```python
from build123d import *

# Parameters (mm, degrees)
SKETCH1_W           = 88.9
SKETCH1_H           = 114.3
BOSS_EXTRUDE1_DEPTH = 5.334
SKETCH2_W           = 5.334
SKETCH2_H           = 16.328571428
CUT_EXTRUDE1_DEPTH  = 6.334
SKETCH2_2_W         = 5.334
SKETCH2_2_H         = 16.328571428
BOSS_EXTRUDE2_DEPTH = 5.334
SKETCH2_3_W         = 5.334
SKETCH2_3_H         = 16.328571428
CUT_EXTRUDE2_DEPTH  = 6.334
CUT_EXTRUDE3_DEPTH  = 6.334


with BuildPart() as part:
    # Sketch1 → Boss-Extrude1 (new body)
    with BuildSketch(Plane(origin=(0, 0, 0), x_dir=(1, 0, 0), z_dir=(0, 1, 0))):
        Rectangle(SKETCH1_W, SKETCH1_H)
    extrude(amount=BOSS_EXTRUDE1_DEPTH)

    # Sketch2 → Cut-Extrude1 (cut, through all)
    with BuildSketch(Plane(origin=(0, 5.334, 0), x_dir=(1, 0, 0), z_dir=(0, 1, 0))):
        with Locations((41.783, -32.657142857)):
            Rectangle(SKETCH2_W, SKETCH2_H)
        with Locations((41.783, 0)):
            Rectangle(SKETCH2_W, SKETCH2_H)
        with Locations((41.783, 32.657142857)):
            Rectangle(SKETCH2_W, SKETCH2_H)
        with Locations((-41.783, 32.657142857)):
            Rectangle(SKETCH2_W, SKETCH2_H)
        with Locations((-41.783, 0)):
            Rectangle(SKETCH2_W, SKETCH2_H)
        with Locations((-41.783, -32.657142857)):
            Rectangle(SKETCH2_W, SKETCH2_H)
    extrude(amount=-CUT_EXTRUDE1_DEPTH, mode=Mode.SUBTRACT)

    # Sketch2_2 → Boss-Extrude2 (add, through all)
    with BuildSketch(Plane(origin=(0, 5.334, 0), x_dir=(1, 0, 0), z_dir=(0, 1, 0))):
        with Locations((41.783, -32.657142857)):
            Rectangle(SKETCH2_2_W, SKETCH2_2_H)
        with Locations((41.783, 0)):
            Rectangle(SKETCH2_2_W, SKETCH2_2_H)
        with Locations((41.783, 32.657142857)):
            Rectangle(SKETCH2_2_W, SKETCH2_2_H)
        with Locations((-41.783, 32.657142857)):
            Rectangle(SKETCH2_2_W, SKETCH2_2_H)
        with Locations((-41.783, 0)):
            Rectangle(SKETCH2_2_W, SKETCH2_2_H)
        with Locations((-41.783, -32.657142857)):
            Rectangle(SKETCH2_2_W, SKETCH2_2_H)
    extrude(amount=-BOSS_EXTRUDE2_DEPTH)

    # Sketch2_3 → Cut-Extrude2 (cut, through all)
    with BuildSketch(Plane(origin=(0, 5.334, 0), x_dir=(1, 0, 0), z_dir=(0, 1, 0))):
        with Locations((41.783, -32.657142857)):
            Rectangle(SKETCH2_3_W, SKETCH2_3_H)
        with Locations((41.783, 0)):
            Rectangle(SKETCH2_3_W, SKETCH2_3_H)
        with Locations((41.783, 32.657142857)):
            Rectangle(SKETCH2_3_W, SKETCH2_3_H)
        with Locations((-41.783, 32.657142857)):
            Rectangle(SKETCH2_3_W, SKETCH2_3_H)
        with Locations((-41.783, 0)):
            Rectangle(SKETCH2_3_W, SKETCH2_3_H)
        with Locations((-41.783, -32.657142857)):
            Rectangle(SKETCH2_3_W, SKETCH2_3_H)
    extrude(amount=-CUT_EXTRUDE2_DEPTH, mode=Mode.SUBTRACT)

    # Sketch3 → Cut-Extrude3 (cut, through all)
    with BuildSketch(Plane(origin=(0, 5.334, 0), x_dir=(1, 0, 0), z_dir=(0, 1, 0))):
        Polygon((44.45, 40.821428571), (-39.116, 40.821428571), (-44.45, 40.821428571), (-44.45, 57.15), (44.45, 57.15), align=None)
    extrude(amount=-CUT_EXTRUDE3_DEPTH, mode=Mode.SUBTRACT)


solid = part.part
```
The listing builds one solid part. Answer for the finished solid, in the listing's coordinates (mm). A direction names the side the tool comes from. Round coordinates to 2 decimals unless told otherwise and drop trailing zeros. Order: outer loops, then holes, each group sorted by start corner. A loop starts at its lowest first (then second) coordinate and runs counter-clockwise, first axis right, second up. Notation, with made-up numbers: (56, -33.5) -> (84, -33.5) arc R26 ccw to (84, -2.5) -> close; hole circle Ø10 at (66.5, -10). An arc over 180 degrees is marked (long way). Answer as CSV lines item,"result".
Q1. For a pull along Z with two mould halves and no side action, classify faces 1 (the flat face through (-1, 3, -40.821)), 2 (the flat face through (42, 3, 24.493)), 3 (the flat face through (44.45, 3, -16)) as +Z half, -Z half, draft (parallel to the pull), parting line (faces both ways), or undercut.
Computed values:
face 1,"-Z half"
face 2,"undercut"
face 3,"draft"
Q2. Which of the six approach directions +Z, -Z, +X, -X, +Y, -Y give full straight-line access (tool end or side, diameter ignored) to faces 4 (the flat face through (-1, 5.334, 7)), 5 (the flat face through (-39.116, 3, 0)), 6 (the flat face through (-1, 3, 57.15)), 7 (the flat face through (42, 3, -8.164)), 8 (the flat face through (-39.116, 3, -33))?
Computed values:
face 4,"+Z, -Z, +X, -X, +Y"
face 5,"-X, +Y, -Y"
face 6,"+Z, +X, -X, +Y, -Y"
face 7,"+X, +Y, -Y"
face 8,"-Z, -X, +Y, -Y"
Q3. Given pin 1 (1.6 mm diameter, centred on y = 3.5, z = 36, fed in from +X); pin 2 (1.6 mm diameter, centred on y = 1.5, z = -2, fed in from -X); pin 3 (1.6 mm diameter, centred on x = 41, y = 2, fed in from -Z), each flat-ended and moving along its own axis, determine where each tip first touches the part or whether it passes through.
Computed values:
pin 1,"stops at x = 39.12"
pin 2,"stops at x = -39.12"
pin 3,"stops at z = -24.49"
Q4. Consider line 1 (X direction, y = 0.75, z = 27.5). Determine where the line is inside the solid, lowest interval first. Write a range as from..to.
Computed values:
line 1,"x = -39.12..39.12"
Q5. A cutting plane is placed at A-A on y = 2.3. Determine the outline of the cut face in (x, z).
Computed values:
outline,"(-44.45, -24.49) -> (-39.12, -24.49) -> (-39.12, -40.82) -> (39.12, -40.82) -> (39.12, -24.49) -> (44.45, -24.49) -> (44.45, -8.16) -> (39.12, -8.16) -> (39.12, 8.16) -> (44.45, 8.16) -> (44.45, 24.49) -> (39.12, 24.49) -> (39.12, 40.82) -> (44.45, 40.82) -> (44.45, 57.15) -> (-44.45, 57.15) -> (-44.45, 40.82) -> (-39.12, 40.82) -> (-39.12, 24.49) -> (-44.45, 24.49) -> (-44.45, 8.16) -> (-39.12, 8.16) -> (-39.12, -8.16) -> (-44.45, -8.16) -> close"
Q6. A cutting plane is placed at B-B on z = -7. Determine the outline of the cut face in (x, y), plus the area to 3 significant figures.
Computed values:
outline,"(-39.12, 0) -> (39.12, 0) -> (39.12, 5.33) -> (-39.12, 5.33) -> close"
area,"417 mm^2"
